```python
from build123d import *

# Parameters (mm, degrees)
BOSS_EXTRUDE1_DEPTH     = 6.4
SKETCH1_3_R             = 15.9
SKETCH1_3_R_2           = 9.55
BOSS_EXTRUDE2_DEPTH     = 12.7
SKETCH1_4_W             = 9.53
SKETCH1_4_H             = 31.8
BOSS_EXTRUDE3_DEPTH     = 25.4
RIB1_REACH              = 63.845
SKETCH6_WALL_W          = 157.046570884
SKETCH6_WALL_H          = 6.4
CUT_EXTRUDE1_DEPTH      = 62.844805764
CUT_EXTRUDE1_DEPTH_BACK = 62.844805764
BOSS_EXTRUDE10_DEPTH    = 9.53
SKETCH9_R               = 9.55
BOSS_EXTRUDE11_DEPTH    = 11.2
SKETCH10_W              = 22.2
SKETCH10_H              = 7.9
CUT_EXTRUDE2_DEPTH      = 8
SKETCH11_R              = 1.725
CUT_EXTRUDE3_DEPTH      = 84.552498467
FILLET1_R               = 0.8


with BuildPart() as part:
    # Sketch1 → Boss-Extrude1 (new body)
    with BuildSketch(Plane(origin=(0, 0, 0), x_dir=(1, 0, 0), z_dir=(0, 1, 0))):
        with BuildLine():
            ThreePointArc((0, -15.9), (-15.9, 0), (0, 15.9))
            Line((0, 15.9), (-44.57, 15.9))
            Line((-44.57, 15.9), (-44.57, -15.9))
            Line((-44.57, -15.9), (0, -15.9))
        make_face()
    extrude(amount=BOSS_EXTRUDE1_DEPTH)

    # Sketch1<3> → Boss-Extrude2 (add)
    with BuildSketch(Plane(origin=(0, 0, 0), x_dir=(1, 0, 0), z_dir=(0, 1, 0))):
        with Locations(Location((0, 0, 0), (0, 0, 270))):
            Circle(SKETCH1_3_R)
        with Locations(Location((0, 0, 0), (0, 0, 270))):
            Circle(SKETCH1_3_R_2, mode=Mode.SUBTRACT)
    extrude(amount=BOSS_EXTRUDE2_DEPTH)

    # Sketch1<4> → Boss-Extrude3 (add)
    with BuildSketch(Plane(origin=(0, 0, 0), x_dir=(1, 0, 0), z_dir=(0, 1, 0))):
        with Locations((-49.335, 0)):
            Rectangle(SKETCH1_4_W, SKETCH1_4_H)
    extrude(amount=BOSS_EXTRUDE3_DEPTH)

    # Sketch6 wall → Rib1 (add, up to next)
    with BuildSketch(Plane(origin=(-30.235, 19.05, 0), x_dir=(-0.914310589726, 0.405013759662, 0), z_dir=(-0.405013759662, -0.914310589726, 0)), mode=Mode.PRIVATE) as rib1_sk1:
        Rectangle(SKETCH6_WALL_W, SKETCH6_WALL_H)
    rib1_tool1 = extrude(rib1_sk1.sketch, amount=RIB1_REACH, mode=Mode.PRIVATE) - part.part
    add(rib1_tool1.solids().sort_by_distance((-30.235, 19.05, 0))[0])

    # Sketch7 → Cut-Extrude1 (cut, two sides)
    with BuildSketch(Plane.XY) as cut_extrude1_sk:
        with BuildLine():
            Line((-44.57, 25.4), (-19.669441159, 10.673850552))
            ThreePointArc((-19.669441159, 10.673850552), (-17.213195922, 10.623662856), (-15.9, 12.7))
            Line((-15.9, 12.7), (-44.57, 25.4))
        make_face()
    extrude(amount=CUT_EXTRUDE1_DEPTH, mode=Mode.SUBTRACT)
    extrude(cut_extrude1_sk.sketch, amount=-CUT_EXTRUDE1_DEPTH_BACK, mode=Mode.SUBTRACT)

    # Sketch8 → Boss-Extrude10 (add)
    with BuildSketch(Plane(origin=(-44.57, 0, 0), x_dir=(0, 0, -1), z_dir=(1, 0, 0))):
        with BuildLine():
            Line((-15.9, 25.4), (15.9, 25.4))
            ThreePointArc((15.9, 25.4), (0, 41.3), (-15.9, 25.4))
        make_face()
    extrude(amount=-BOSS_EXTRUDE10_DEPTH)

    # Sketch9 → Boss-Extrude11 (add)
    with BuildSketch(Plane.ZY.offset(54.1)):
        with Locations((0, 25.4)):
            Circle(SKETCH9_R)
    extrude(amount=BOSS_EXTRUDE11_DEPTH)

    # Sketch10 → Cut-Extrude2 (cut)
    with BuildSketch(Plane.ZY.offset(54.1)):
        with Locations((0, 10.25)):
            Rectangle(SKETCH10_W, SKETCH10_H)
    extrude(amount=-CUT_EXTRUDE2_DEPTH, mode=Mode.SUBTRACT)

    # Sketch11 → Cut-Extrude3 (cut, through all)
    with BuildSketch(Plane.XY.offset(15.9)):
        with Locations((-50.9, 10.3)):
            Circle(SKETCH11_R)
    extrude(amount=-CUT_EXTRUDE3_DEPTH, mode=Mode.SUBTRACT)

    # Fillet1
    fillet1_edges = [part.edges().sort_by_distance(p)[0] for p in [
        (-46.1, 10.25, -11.1),
        (-50.1, 6.3, -11.1),
        (-46.1, 14.2, 0),
        (-50.1, 14.2, -11.1),
        (-46.1, 10.25, 11.1),
        (-50.1, 14.2, 11.1),
        (-46.1, 6.3, 0),
        (-50.1, 6.3, 11.1),
        (-44.57, 15.9, 3.2),
        (-30.072329452, 6.4, 3.2),
        (-44.57, 15.9, -3.2),
        (-30.072329452, 6.4, -3.2),
    ]]
    fillet(fillet1_edges, radius=FILLET1_R)


solid = part.part
```
Input: part model. Units: mm. Frame: model coordinates. A direction names the side the tool comes from. Coordinates: 2 decimals unless noted, no trailing zeros. Write each loop counter-clockwise with the first axis right and the second up, starting at its lowest first coordinate (ties: lowest second). Pieces come first, ordered by that corner, then holes. Notation, with made-up numbers: (-28, 84.25) - (18, 84.25) arc R32 cw to (18, 111.25) - close; hole circle Ø1 at (-33, 86.5). An arc over 180 degrees is marked (long way). Put each result on its own line as item: value. Start each with the question number.
1) Reachability of faces 1 (the face through (-28, 6.4, 10)), 2 (the face through (-7, 12.7, 7)), 3 (the face through (-46.1, 10, 0)) from +Z, -Z, +X, -X, +Y, -Y: full face, straight path, thin tool, end or side. Return the list, or none.
2) Ray query, L1, parallel to X at y = 3.5, z = 0; L2, parallel to X at y = 32.5, z = -8.5; L3, parallel to Y at x = -27, z = 7.5. Return the intervals inside material, ascending.
3) Mould query, pull axis Z, two halves, no side actions, for faces 4 (the face through (-34, 14, 3.2)), 5 (the face through (-49, 10, 11.1)), 6 (the face through (-54.1, 16, 4)), 7 (the face through (-49.268, 41.296, -0.35)). Classes: pulls with the +Z half, pulls with the -Z half, needs draft (parallel to the pull), parting line crosses it, or undercut.
4) Cut plane D-D (y = 19). Return the cut outline in (x, z), plus the area to 3 significant figures.
5) Cut plane B-B (z = -2). Return the cut outline in (x, y).
6) Cut plane C-C (y = 5.5). Return the cut outline in (x, z).
7) Cut plane A-A (x = -50.9). Return the cut outline in (y, z) (3 decimals).
8) Contact query for flat-ended pins moving along their axis: pin 1 (6 mm diameter, centred on x = -12, z = -8, fed in from +Y); pin 2 (12 mm diameter, centred on x = -36, z = 11.5, fed in from +Y); pin 3 (7 mm diameter, centred on y = 10.5, z = 0.5, fed in from -X). Output: stop coordinate, or through.
Resolved:
1. face 1: +Z, +Y
1. face 2: +Z, -Z, +X, +Y
1. face 3: -X
2. L1: x = -54.1 to -9.55, 9.55 to 15.9
2. L2: x = -54.1 to -44.57
2. L3: y = 0 to 6.4
3. face 4: pulls with the +Z half
3. face 5: undercut
3. face 6: needs draft
3. face 7: parting line crosses it
4. outline: (-65.3, -7.09) - (-54.1, -7.09) - (-54.1, -15.9) - (-44.57, -15.9) - (-44.57, -4) arc R0.8 cw to (-43.77, -3.2) - (-33.75, -3.2) - (-33.75, 3.2) - (-43.77, 3.2) arc R0.8 cw to (-44.57, 4) - (-44.57, 15.9) - (-54.1, 15.9) - (-54.1, 7.09) - (-65.3, 7.09) - close
4. area: 531 mm2
5. outline: (-65.3, 16.06) - (-54.1, 16.06) - (-54.1, 14.2) - (-46.9, 14.2) arc R0.8 cw to (-46.1, 13.4) - (-46.1, 7.1) arc R0.8 cw to (-46.9, 6.3) - (-54.1, 6.3) - (-54.1, 0) - (-9.34, 0) - (-9.34, 12.7) - (-15.77, 12.7) - (-15.77, 12.64) - (-15.9, 12.7) arc R2.5 cw to (-19.67, 10.67) - (-44.57, 25.4) - (-44.57, 41.17) - (-54.1, 41.17) - (-54.1, 34.74) - (-65.3, 34.74) - close; (9.34, 0) - (15.77, 0) - (15.77, 12.7) - (9.34, 12.7) - close
6. outline: (-54.1, -15.9) - (0, -15.9) arc R15.9 ccw to (0, 15.9) - (-54.1, 15.9) - close; hole circle Ø19.1 at (0, 0)
7. outline: (0, -15.9) - (8.575, -15.9) - (8.575, -11.1) - (7.1, -11.1) arc R0.8 cw to (6.3, -10.3) - (6.3, 10.3) arc R0.8 cw to (7.1, 11.1) - (8.575, 11.1) - (8.575, 15.9) - (0, 15.9) - close; (12.025, -15.9) - (25.4, -15.9) arc R15.9 ccw to (25.4, 15.9) - (12.025, 15.9) - (12.025, 11.1) - (13.4, 11.1) arc R0.8 cw to (14.2, 10.3) - (14.2, -10.3) arc R0.8 cw to (13.4, -11.1) - (12.025, -11.1) - close
8. pin 1: stops at y = 12.7
8. pin 2: stops at y = 6.4
8. pin 3: stops at x = -46.37
